from build123d import *

# Parameters (mm, degrees)
SKETCH5_R           = 2.5
SKETCH5_R_2         = 52.3875
SKETCH5_R_3         = 4.5
SKETCH5_R_4         = 27.4955
BOSS_EXTRUDE2_DEPTH = 7.62
CUT_EXTRUDE1_REACH  = 239.718
SKETCH7_R           = 3.302
CUT_EXTRUDE2_REACH  = 239.718
FILLET1_R           = 6.35
CUT_EXTRUDE18_REACH = 239.718
CUT_EXTRUDE22_REACH = 239.718
CUT_EXTRUDE23_REACH = 239.718
CUT_EXTRUDE24_REACH = 239.718
FILLET2_R           = 6.35


with BuildPart() as part:
    # Sketch5 → Boss-Extrude2 (new body)
    with BuildSketch(Plane(origin=(0, 0, 0), x_dir=(-1, 0, 0), z_dir=(0, 1, 0))):
        with BuildLine():
            ThreePointArc((-65.654330467, 67.1325302), (-87.334586589, 76.112786321), (-78.354330467, 54.4325302))
            Line((-78.354330467, 54.4325302), (-78.354330467, -65.2014698))
            ThreePointArc((-78.354330467, -65.2014698), (-87.334586589, -86.881725921), (-65.654330467, -77.9014698))
            ThreePointArc((-65.654330467, -77.9014698), (-61.934586589, -68.921213679), (-52.954330467, -65.2014698))
            Line((-52.954330467, -65.2014698), (124.845669533, -65.2014698))
            ThreePointArc((124.845669533, -65.2014698), (133.825925654, -68.921213679), (137.545669533, -77.9014698))
            ThreePointArc((137.545669533, -77.9014698), (159.225925654, -86.881725921), (150.245669533, -65.2014698))
            Line((150.245669533, -65.2014698), (171.77131, 3.1242))
            ThreePointArc((171.77131, 3.1242), (215.601286514, 35.222255536), (198.228973896, 86.696081552))
            ThreePointArc((198.228973896, 86.696081552), (196.548809881, 87.149442365), (194.971173285, 86.414901751))
            Line((194.971173285, 86.414901751), (189.706289667, 81.150018133))
            ThreePointArc((189.706289667, 81.150018133), (182.622653279, 79.740995249), (178.61009559, 85.746212211))
            Line((178.61009559, 85.746212211), (178.61009559, 92.318945001))
            ThreePointArc((178.61009559, 92.318945001), (177.952930296, 94.023800851), (176.32148656, 94.846473949))
            ThreePointArc((176.32148656, 94.846473949), (171.77131, 95.0722), (167.22113344, 94.846473949))
            ThreePointArc((167.22113344, 94.846473949), (165.589689704, 94.023800851), (164.93252441, 92.318945001))
            Line((164.93252441, 92.318945001), (164.93252441, 85.746212211))
            ThreePointArc((164.93252441, 85.746212211), (158.43252441, 79.246212211), (151.93252441, 85.746212211))
            Line((151.93252441, 85.746212211), (151.93252441, 86.323222653))
            ThreePointArc((151.93252441, 86.323222653), (150.643024247, 88.534070942), (148.083823499, 88.500124563))
            Line((148.083823499, 88.500124563), (0, 61.9125))
            Line((0, 61.9125), (-65.654330467, 67.1325302))
        make_face()
        with Locations(Location((0, -57.15, 0), (0, 0, 90))):
            Circle(SKETCH5_R, mode=Mode.SUBTRACT)
        with Locations(Location((-57.15, 0, 0), (0, 0, 90))):
            Circle(SKETCH5_R, mode=Mode.SUBTRACT)
        with Locations(Location((0, 0, 0), (0, 0, 90))):
            Circle(SKETCH5_R_2, mode=Mode.SUBTRACT)
        with Locations(Location((57.15, 0, 0), (0, 0, 90))):
            Circle(SKETCH5_R, mode=Mode.SUBTRACT)
        with Locations(Location((158.432556474, 12.450347008, 0), (0, 0, 90))):
            Circle(SKETCH5_R_3, mode=Mode.SUBTRACT)
        with Locations(Location((185.110017809, 12.450330368, 0), (0, 0, 90))):
            Circle(SKETCH5_R_3, mode=Mode.SUBTRACT)
        with Locations(Location((0, 57.15, 0), (0, 0, 90))):
            Circle(SKETCH5_R, mode=Mode.SUBTRACT)
        with Locations(Location((137.996446159, 29.598301358, 0), (0, 0, 90))):
            Circle(SKETCH5_R_3, mode=Mode.SUBTRACT)
        with Locations(Location((205.546149516, 29.598259225, 0), (0, 0, 90))):
            Circle(SKETCH5_R_3, mode=Mode.SUBTRACT)
        with Locations(Location((171.77131, 49.0982, 0), (0, 0, 90))):
            Circle(SKETCH5_R_4, mode=Mode.SUBTRACT)
        with Locations(Location((133.36397, 55.870475, 0), (0, 0, 90))):
            Circle(SKETCH5_R_3, mode=Mode.SUBTRACT)
        with Locations(Location((210.178658448, 55.870427088, 0), (0, 0, 90))):
            Circle(SKETCH5_R_3, mode=Mode.SUBTRACT)
        with Locations(Location((146.702715077, 78.973825904, 0), (0, 0, 90))):
            Circle(SKETCH5_R_3, mode=Mode.SUBTRACT)
        with Locations(Location((171.771334325, 88.098039417, 0), (0, 0, 90))):
            Circle(SKETCH5_R_3, mode=Mode.SUBTRACT)
        with Locations(Location((196.839942191, 78.973794632, 0), (0, 0, 90))):
            Circle(SKETCH5_R_3, mode=Mode.SUBTRACT)
    extrude(amount=BOSS_EXTRUDE2_DEPTH)

    # Sketch7 → Cut-Extrude1 (cut, up to next)
    with BuildSketch(Plane(origin=(0, 7.62, 0), x_dir=(1, 0, 0), z_dir=(0, 1, 0)), mode=Mode.PRIVATE) as cut_extrude1_sk1:
        with Locations(Location((78.354330467, 77.9014698, 0), (0, 0, 270))):
            Circle(SKETCH7_R)
    cut_extrude1_tool1 = extrude(cut_extrude1_sk1.sketch, amount=-CUT_EXTRUDE1_REACH, mode=Mode.PRIVATE) & part.part
    # Sketch7 → Cut-Extrude1 (cut, up to next)
    with BuildSketch(Plane(origin=(0, 7.62, 0), x_dir=(1, 0, 0), z_dir=(0, 1, 0)), mode=Mode.PRIVATE) as cut_extrude1_sk2:
        with Locations(Location((78.354330467, -67.1325302, 0), (0, 0, 270))):
            Circle(SKETCH7_R)
    cut_extrude1_tool2 = extrude(cut_extrude1_sk2.sketch, amount=-CUT_EXTRUDE1_REACH, mode=Mode.PRIVATE) & part.part
    # Sketch7 → Cut-Extrude1 (cut, up to next)
    with BuildSketch(Plane(origin=(0, 7.62, 0), x_dir=(1, 0, 0), z_dir=(0, 1, 0)), mode=Mode.PRIVATE) as cut_extrude1_sk3:
        with Locations(Location((-150.245669533, 77.9014698, 0), (0, 0, 270))):
            Circle(SKETCH7_R)
    cut_extrude1_tool3 = extrude(cut_extrude1_sk3.sketch, amount=-CUT_EXTRUDE1_REACH, mode=Mode.PRIVATE) & part.part
    add(cut_extrude1_tool1.solids().sort_by_distance((78.35433, 7.62, -77.90147))[0], mode=Mode.SUBTRACT)
    add(cut_extrude1_tool2.solids().sort_by_distance((78.35433, 7.62, 67.13253))[0], mode=Mode.SUBTRACT)
    add(cut_extrude1_tool3.solids().sort_by_distance((-150.24567, 7.62, -77.90147))[0], mode=Mode.SUBTRACT)

    # Sketch9 → Cut-Extrude2 (cut, up to next)
    with BuildSketch(Plane(origin=(0, 7.62, 0), x_dir=(1, 0, 0), z_dir=(0, 1, 0)), mode=Mode.PRIVATE) as cut_extrude2_sk1:
        with BuildLine():
            Line((78.354330467, -54.4325302), (65.479533423, -1.373188973))
            ThreePointArc((65.479533423, -1.373188973), (65.301620926, 0.002964909), (65.426874021, 1.384907029))
            Line((65.426874021, 1.384907029), (78.354330467, 65.2014698))
            Line((78.354330467, 65.2014698), (78.354330467, -54.4325302))
        make_face()
    cut_extrude2_tool1 = extrude(cut_extrude2_sk1.sketch, amount=-CUT_EXTRUDE2_REACH, mode=Mode.PRIVATE) & part.part
    add(cut_extrude2_tool1.solids().sort_by_distance((73.953245, 7.62, -3.5903))[0], mode=Mode.SUBTRACT)

    # Fillet1
    fillet1_edges = [part.edges().sort_by_distance(p)[0] for p in [
        (78.354330467, 3.81, -65.2014698),
        (78.354330467, 3.81, 54.4325302),
    ]]
    fillet(fillet1_edges, radius=FILLET1_R)

    # Sketch18 → Cut-Extrude18 (cut, up to next)
    with BuildSketch(Plane(origin=(0, 7.62, 0), x_dir=(1, 0, 0), z_dir=(0, 1, 0)), mode=Mode.PRIVATE) as cut_extrude18_sk1:
        with BuildLine():
            Line((0, -61.9125), (-127.619272771, -61.9125))
            ThreePointArc((-127.619272771, -61.9125), (-135.339514958, -77.139829518), (-148.083823499, -88.500124563))
            Line((-148.083823499, -88.500124563), (0, -61.9125))
        make_face()
    cut_extrude18_tool1 = extrude(cut_extrude18_sk1.sketch, amount=-CUT_EXTRUDE18_REACH, mode=Mode.PRIVATE) & part.part
    add(cut_extrude18_tool1.solids().sort_by_distance((-89.926243, 7.62, 70.546245))[0], mode=Mode.SUBTRACT)

    # Sketch23 → Cut-Extrude22 (cut, up to next)
    with BuildSketch(Plane(origin=(0, 7.62, 0), x_dir=(1, 0, 0), z_dir=(0, 1, 0)), mode=Mode.PRIVATE) as cut_extrude22_sk1:
        with BuildLine():
            Line((44.404686705, 47.70167394), (49.357095568, 39.22528171))
            ThreePointArc((49.357095568, 39.22528171), (54.839881255, 36.078648861), (60.322666943, 39.22528171))
            Line((60.322666943, 39.22528171), (65.275075806, 47.70167394))
            ThreePointArc((65.275075806, 47.70167394), (65.299734236, 54.065825692), (59.792290118, 57.255041091))
            Line((59.792290118, 57.255041091), (49.887472392, 57.255041091))
            ThreePointArc((49.887472392, 57.255041091), (44.380028275, 54.065825692), (44.404686705, 47.70167394))
        make_face()
    cut_extrude22_tool1 = extrude(cut_extrude22_sk1.sketch, amount=-CUT_EXTRUDE22_REACH, mode=Mode.PRIVATE) & part.part
    add(cut_extrude22_tool1.solids().sort_by_distance((54.839881, 7.62, -48.088951))[0], mode=Mode.SUBTRACT)

    # Sketch24 → Cut-Extrude23 (cut, up to next)
    with BuildSketch(Plane(origin=(0, 7.62, 0), x_dir=(1, 0, 0), z_dir=(0, 1, 0)), mode=Mode.PRIVATE) as cut_extrude23_sk1:
        with BuildLine():
            Line((-128.021835855, -9.473541553), (-128.021835855, -47.532808157))
            ThreePointArc((-128.021835855, -47.532808157), (-126.087569038, -52.20254134), (-121.417835855, -54.136808157))
            Line((-121.417835855, -54.136808157), (-49.347167305, -54.136808157))
            ThreePointArc((-49.347167305, -54.136808157), (-43.269796158, -50.117063552), (-44.590813829, -42.951332672))
            ThreePointArc((-44.590813829, -42.951332672), (-55.149477043, -28.13703677), (-60.946622173, -10.89343389))
            ThreePointArc((-60.946622173, -10.89343389), (-63.208539256, -6.9914866), (-67.447595205, -5.451400172))
            Line((-67.447595205, -5.451400172), (-123.999694474, -5.451400172))
            ThreePointArc((-123.999694474, -5.451400172), (-126.843777919, -6.629458107), (-128.021835855, -9.473541553))
        make_face()
    cut_extrude23_tool1 = extrude(cut_extrude23_sk1.sketch, amount=-CUT_EXTRUDE23_REACH, mode=Mode.PRIVATE) & part.part
    # Sketch24 → Cut-Extrude23 (cut, up to next)
    with BuildSketch(Plane(origin=(0, 7.62, 0), x_dir=(1, 0, 0), z_dir=(0, 1, 0)), mode=Mode.PRIVATE) as cut_extrude23_sk2:
        with BuildLine():
            Line((-48.030119475, 55.467262227), (-133.757395028, 55.467262227))
            ThreePointArc((-133.757395028, 55.467262227), (-140.91596397, 53.199285335), (-145.462549697, 47.222882847))
            Line((-145.462549697, 47.222882847), (-154.629174486, 21.597614724))
            ThreePointArc((-154.629174486, 21.597614724), (-153.087569165, 10.251898923), (-142.924019817, 4.978941625))
            Line((-142.924019817, 4.978941625), (-67.530335669, 4.978941625))
            ThreePointArc((-67.530335669, 4.978941625), (-63.273580756, 6.533896803), (-61.021387653, 10.466513517))
            ThreePointArc((-61.021387653, 10.466513517), (-54.860712254, 28.695991135), (-43.400710369, 44.153550205))
            ThreePointArc((-43.400710369, 44.153550205), (-41.918010421, 51.364249812), (-48.030119475, 55.467262227))
        make_face()
    cut_extrude23_tool2 = extrude(cut_extrude23_sk2.sketch, amount=-CUT_EXTRUDE23_REACH, mode=Mode.PRIVATE) & part.part
    add(cut_extrude23_tool1.solids().sort_by_distance((-90.134227, 7.62, 31.015027))[0], mode=Mode.SUBTRACT)
    add(cut_extrude23_tool2.solids().sort_by_distance((-101.091436, 7.62, -30.758334))[0], mode=Mode.SUBTRACT)

    # Sketch25 → Cut-Extrude24 (cut, up to next)
    with BuildSketch(Plane(origin=(0, 7.62, 0), x_dir=(1, 0, 0), z_dir=(0, 1, 0)), mode=Mode.PRIVATE) as cut_extrude24_sk1:
        with BuildLine():
            Line((77.350104134, -50.293933877), (65.301620926, 0.002964909))
            Line((65.301620926, 0.002964909), (65.301620926, -42.8625))
            ThreePointArc((65.301620926, -42.8625), (51.831236744, -48.442115818), (46.251620926, -61.9125))
            Line((46.251620926, -61.9125), (0, -61.9125))
            Line((0, -61.9125), (65.654330467, -67.1325302))
            ThreePointArc((65.654330467, -67.1325302), (86.020660704, -77.257616901), (81.798799869, -54.908552511))
            ThreePointArc((81.798799869, -54.908552511), (78.949471352, -53.203752084), (77.350104134, -50.293933877))
        make_face()
    cut_extrude24_tool1 = extrude(cut_extrude24_sk1.sketch, amount=-CUT_EXTRUDE24_REACH, mode=Mode.PRIVATE) & part.part
    add(cut_extrude24_tool1.solids().sort_by_distance((67.004182, 7.62, 55.543005))[0], mode=Mode.SUBTRACT)

    # Fillet2
    fillet2_edges = [part.edges().sort_by_distance(p)[0] for p in [
        (65.301620926, 3.81, 42.8625),
        (46.251620926, 3.81, 61.9125),
    ]]
    fillet(fillet2_edges, radius=FILLET2_R)


solid = part.part
Part model, mm, in its own coordinate system. A direction names the side the tool comes from. Coordinates: 2 decimals unless noted, no trailing zeros. Use a Markdown table: item, result. Add a question column.
Item 1: Probe probe 1 along X at (y, z) = (2.5, -78); probe 2 along X at (y, z) = (7, 41.5); probe 3 along Z at (x, y) = (-92, 3.75). List the from-to ranges inside material, lowest first.
Item 2: Band-saw the part on A-A on y = 2.25. Give the number of separate pieces and of enclosed holes in the cut face, plus the area to 3 significant figures.
Item 3: Which spindle directions (+Z, -Z, +X, -X, +Y, -Y) get a long thin tool onto all of the face, cutting with end or side? Do faces 4 (the flat face through (-160.858, 3.757, -31.517)), 5 (the flat face through (-74, 0, 3)), 6 (the cylindrical face through (-54.986, 3.863, -28.456)). Say none if no direction does.
Item 4: Pull direction Z, two halves, no side cores. Call faces 1 (the cylindrical face through (51.932, 3.863, 48.342)), 2 (the cylindrical face through (-43.313, 3.863, 50.216)), 3 (the flat face through (-164.933, 4, 89)): +Z half, -Z half, draft (parallel to the pull), parting line (faces both ways), or undercut.
Item 5: Flat gauge pins, fed straight in: P1, Ø10.5, axis at x = -158.43, z = 12.45, coming from the -Y side; P2, Ø4, axis at x = -46.5, y = 3.5, coming from the -Z side; P3, Ø7, axis at x = -205.55, z = 29.6, coming from the +Y side; P4, Ø1, axis at x = -34.5, y = 4, coming from the +Z side. Where does each tip first touch, or does it go through?
Geometry says:
| question | item | result |
|---|---|---|
| 1 | probe 1 | -162.95 to -153.55, -146.95 to -137.55, 65.65 to 75.05, 81.65 to 91.05 |
| 1 | probe 2 | -217.11 to -198.2, -145.35 to -128.02, -45.94 to -31.97, 31.97 to 63.73 |
| 1 | probe 3 | -65.2 to -55.47, -4.98 to 5.45, 54.14 to 61.91 |
| 2 | separate pieces | 1 |
| 2 | enclosed holes | 20 |
| 2 | area | 14,100 mm² |
| 3 | face 4 | -X, +Y, -Y |
| 3 | face 5 | +Z, -Z, +X, -X, -Y |
| 3 | face 6 | +Y, -Y |
| 4 | face 1 | +Z half |
| 4 | face 2 | undercut |
| 4 | face 3 | draft |
| 5 | P1 | y = 0 |
| 5 | P2 | z = -65.2 |
| 5 | P3 | through |
| 5 | P4 | z = 61.91 |
